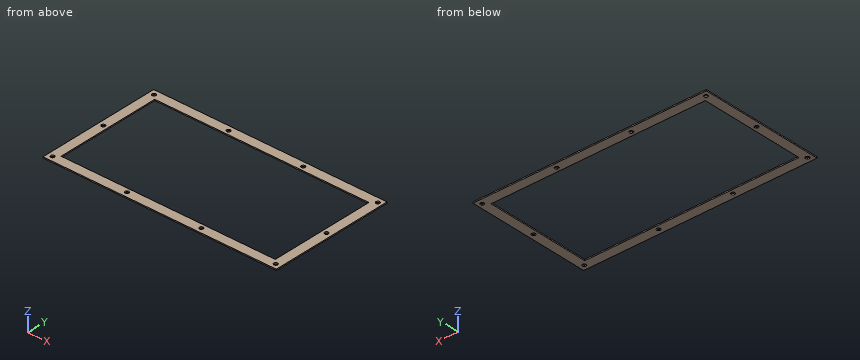
```python
from build123d import *

# Parameters (mm, degrees)
SKETCH1_W           = 610
SKETCH1_H           = 325
SKETCH1_W_2         = 560
SKETCH1_H_2         = 275
BOSS_EXTRUDE1_DEPTH = 3
SKETCH2_R           = 5
CUT_EXTRUDE1_DEPTH  = 4
LPATTERN1_COUNT     = 4
LPATTERN1_PITCH     = 195
LPATTERN2_COUNT     = 3
LPATTERN2_PITCH     = 149
LPATTERN3_OUTLINE_R = 5
LPATTERN3_DEPTH     = 3
LPATTERN4_OUTLINE_R = 5
LPATTERN4_DEPTH     = 3


# Read off the part's stored shape, not the designer's step: LPattern3, LPattern4
with BuildPart() as part:
    # Sketch1 → Boss-Extrude1 (new body)
    with BuildSketch(Plane.XY):
        with Locations((-100, -37.5)):
            Rectangle(SKETCH1_W, SKETCH1_H)
        with Locations((-100, -37.5)):
            Rectangle(SKETCH1_W_2, SKETCH1_H_2, mode=Mode.SUBTRACT)
    extrude(amount=BOSS_EXTRUDE1_DEPTH)

    # Sketch2 → Cut-Extrude1 (cut)
    with BuildSketch(Plane.XY.offset(3)):
        with Locations((-392, 111.5)):
            Circle(SKETCH2_R)
    cut_extrude1 = extrude(amount=-CUT_EXTRUDE1_DEPTH, mode=Mode.SUBTRACT)

    # LPattern1: Cut-Extrude1 ×4
    with Locations(*[(i * LPATTERN1_PITCH, 0, 0) for i in range(1, LPATTERN1_COUNT)]):
        add(cut_extrude1, mode=Mode.SUBTRACT)

    # LPattern2: Cut-Extrude1 ×3
    with Locations(*[(0, -i * LPATTERN2_PITCH, 0) for i in range(1, LPATTERN2_COUNT)]):
        add(cut_extrude1, mode=Mode.SUBTRACT)

    # LPattern3 outline → LPattern3 (cut)
    with BuildSketch(Plane.XY):
        with Locations((191.5, -186.5)):
            Circle(LPATTERN3_OUTLINE_R)
        with Locations((-3, -186.5)):
            Circle(LPATTERN3_OUTLINE_R)
        with Locations((-197.5, -186.5)):
            Circle(LPATTERN3_OUTLINE_R)
    extrude(amount=LPATTERN3_DEPTH, mode=Mode.SUBTRACT)

    # LPattern4 outline → LPattern4 (cut)
    with BuildSketch(Plane.XY):
        with Locations((191.5, -37.5)):
            Circle(LPATTERN4_OUTLINE_R)
    extrude(amount=LPATTERN4_DEPTH, mode=Mode.SUBTRACT)


solid = part.part
```
CAD build for the part. Positions are in the model's coordinates, mm. Round coordinates to 2 decimals unless told otherwise and drop trailing zeros. Order: outer loops, then holes, each group sorted by start corner. A loop starts at its lowest first (then second) coordinate and runs counter-clockwise, first axis right, second up. Notation, with made-up numbers: (52.5, 33) - (83.5, 33) arc R26 cw to (83.5, 72) - close; hole circle Ø1 at (39, -18). An arc over 180 degrees is marked (long way). Answer in a Markdown table with one row per item. Add a question column.
(1) Band-saw the part on C-C on z = 1.7. Count the separate pieces of the cut face and the enclosed holes in it, and give its area (3 significant figures).
(2) Band-saw the part on B-B on x = -266. List the corners of the cut face in (y, z).
(3) Probe L1, parallel to X at y = 12.5, z = 0.85; L2, parallel to Y at x = -108.5, z = 2.2; L3, parallel to Y at x = -2, z = 1.6. List the from-to ranges inside material, lowest first. Write a range as [from, to].
(4) Band-saw the part on A-A on y = 39.5. List the corners of the cut face in (x, z), and give its area (3 significant figures).
Data:
| question | item | result |
|---|---|---|
| 1 | separate pieces | 1 |
| 1 | enclosed holes | 11 |
| 1 | area | 43,500 mm^2 |
| 2 | outline | (-200, 0) - (-175, 0) - (-175, 3) - (-200, 3) - close; (100, 0) - (125, 0) - (125, 3) - (100, 3) - close |
| 3 | L1 | x = [-405, -380], [180, 205] |
| 3 | L2 | y = [-200, -175], [100, 125] |
| 3 | L3 | y = [-200, -191.4], [-181.6, -175], [100, 106.5], [116.5, 125] |
| 4 | outline | (-405, 0) - (-380, 0) - (-380, 3) - (-405, 3) - close; (180, 0) - (205, 0) - (205, 3) - (180, 3) - close |
| 4 | area | 150 mm^2 |
